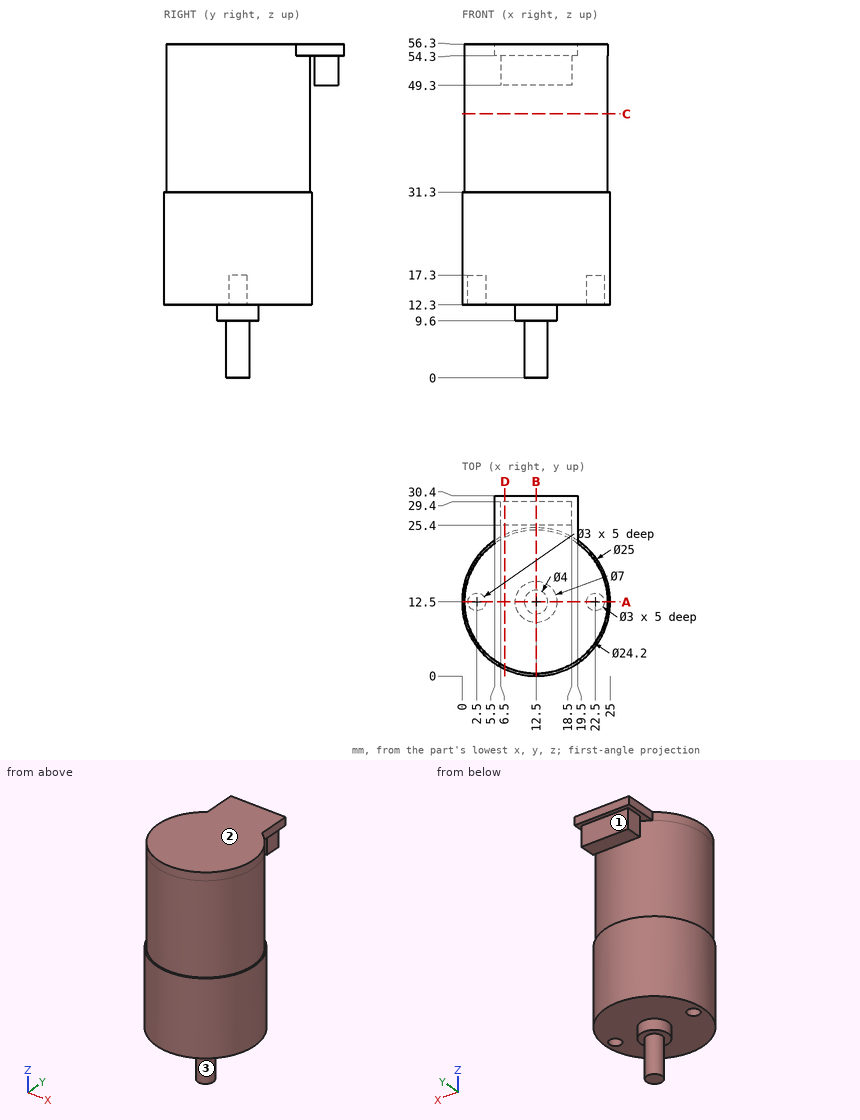
Geometry check sheet. Reference: drawing and pictorial views, mm from the part's lowest x, y, z. A direction names the side the tool comes from. Coordinates: 2 decimals unless noted, no trailing zeros. Write each loop counter-clockwise with the first axis right and the second up, starting at its lowest first coordinate (ties: lowest second). Pieces come first, ordered by that corner, then holes.
Item 1: Depth check by flat-ended pin: pin 1 Ø5 at (y, z) = (5, 10.5) entering from +X; pin 2 Ø8 at (x, z) = (6, 24.5) entering from +Y; pin 3 Ø8 at (x, y) = (12, 26.5) entering from -Z. Enter the tip coordinate at first touch or a pass-through.
Numbers:
pin 1: stops at x = 23.59
pin 2: stops at y = 24.75
pin 3: stops at z = 12.3
Item 2: Cross-section at A-A on y = 12.5. Record the boundary of the cut face in (x, z), then the cut area to 3 significant figures.
Numbers:
outline: (0, 12.3) - (1, 12.3) - (1, 17.3) - (4, 17.3) - (4, 12.3) - (9, 12.3) - (9, 9.6) - (10.5, 9.6) - (10.5, 0) - (14.5, 0) - (14.5, 9.6) - (16, 9.6) - (16, 12.3) - (21, 12.3) - (21, 17.3) - (24, 17.3) - (24, 12.3) - (25, 12.3) - (25, 31.3) - (24.6, 31.3) - (24.6, 56.3) - (0.4, 56.3) - (0.4, 31.3) - (0, 31.3) - close
area: 1,110 mm2
Item 3: Cross-section at D-D on x = 7.25. Record the boundary of the cut face in (y, z).
Numbers:
outline: (1.16, 12.3) - (23.84, 12.3) - (23.84, 31.3) - (23.4, 31.3) - (23.4, 54.3) - (25.4, 54.3) - (25.4, 49.3) - (29.4, 49.3) - (29.4, 54.3) - (30.4, 54.3) - (30.4, 56.3) - (1.6, 56.3) - (1.6, 31.3) - (1.16, 31.3) - close
Item 4: Cross-section at B-B on x = 12.5. Record the boundary of the cut face in (y, z).
Numbers:
outline: (0, 12.3) - (9, 12.3) - (9, 9.6) - (10.5, 9.6) - (10.5, 0) - (14.5, 0) - (14.5, 9.6) - (16, 9.6) - (16, 12.3) - (25, 12.3) - (25, 31.3) - (24.6, 31.3) - (24.6, 54.3) - (25.4, 54.3) - (25.4, 49.3) - (29.4, 49.3) - (29.4, 54.3) - (30.4, 54.3) - (30.4, 56.3) - (0.4, 56.3) - (0.4, 31.3) - (0, 31.3) - close
Item 5: Access from +Z, -Z, +X, -X, +Y, -Y to the whole of each face (thin tool, end or side, straight path). Record for the marked faces 1, 2 and 3.
Numbers:
face 1: -Z, +X, -X, +Y
face 2: +Z, +X, -X, +Y, -Y
face 3: -Z
Item 6: Scan lines: probe 1 along X at (y, z) = (12, 15); probe 2 along Y at (x, z) = (12.5, 39); probe 3 along Z at (x, y) = (3.5, 21). Record each from-to range of solid material in increasing order.
Numbers:
probe 1: x = 0.01 to 1.09, 3.91 to 21.09, 23.91 to 24.99
probe 2: y = 0.4 to 24.6
probe 3: z = 12.3 to 31.3
Item 7: Cross-section at C-C on z = 44.5. Record the boundary of the cut face in (x, y).
Numbers:
outline: circle Ø24.2 at (12.5, 12.5)
